```python
from build123d import *

# Parameters (mm, degrees)
SKETCH1_W           = 250
SKETCH1_H           = 62.9
BOSS_EXTRUDE1_DEPTH = 3
SKETCH3_W           = 3
SKETCH3_H           = 20
CUT_EXTRUDE1_DEPTH  = 258.808863308
CUT_EXTRUDE2_REACH  = 259.809
SKETCH4_W           = 20
SKETCH4_H           = 3
CUT_EXTRUDE3_REACH  = 259.809
SKETCH5_W           = 20
SKETCH5_H           = 3
CUT_EXTRUDE4_REACH  = 259.809
SKETCH6_W           = 90
SKETCH6_H           = 3


with BuildPart() as part:
    # Sketch1 → Boss-Extrude1 (new body)
    with BuildSketch(Plane(origin=(0, 0, 0), x_dir=(1, 0, 0), z_dir=(0, 1, 0))):
        with Locations((125, 31.45)):
            Rectangle(SKETCH1_W, SKETCH1_H)
    extrude(amount=BOSS_EXTRUDE1_DEPTH)

    # Sketch3 → Cut-Extrude1 (cut, through all)
    with BuildSketch(Plane(origin=(0, 3, 0), x_dir=(1, 0, 0), z_dir=(0, 1, 0))):
        with Locations((1.5, 32.9)):
            Rectangle(SKETCH3_W, SKETCH3_H)
        with Locations((248.5, 32.9)):
            Rectangle(SKETCH3_W, SKETCH3_H)
    extrude(amount=-CUT_EXTRUDE1_DEPTH, mode=Mode.SUBTRACT)

    # Sketch4 → Cut-Extrude2 (cut, up to next)
    with BuildSketch(Plane(origin=(0, 3, 0), x_dir=(1, 0, 0), z_dir=(0, 1, 0)), mode=Mode.PRIVATE) as cut_extrude2_sk1:
        with Locations((10, 61.4)):
            Rectangle(SKETCH4_W, SKETCH4_H)
    cut_extrude2_tool1 = extrude(cut_extrude2_sk1.sketch, amount=-CUT_EXTRUDE2_REACH, mode=Mode.PRIVATE) & part.part
    add(cut_extrude2_tool1.solids().sort_by_distance((10, 3, -61.4))[0], mode=Mode.SUBTRACT)

    # Sketch5 → Cut-Extrude3 (cut, up to next)
    with BuildSketch(Plane(origin=(0, 3, 0), x_dir=(1, 0, 0), z_dir=(0, 1, 0)), mode=Mode.PRIVATE) as cut_extrude3_sk1:
        with Locations((240, 61.4)):
            Rectangle(SKETCH5_W, SKETCH5_H)
    cut_extrude3_tool1 = extrude(cut_extrude3_sk1.sketch, amount=-CUT_EXTRUDE3_REACH, mode=Mode.PRIVATE) & part.part
    add(cut_extrude3_tool1.solids().sort_by_distance((240, 3, -61.4))[0], mode=Mode.SUBTRACT)

    # Sketch6 → Cut-Extrude4 (cut, up to next)
    with BuildSketch(Plane(origin=(0, 3, 0), x_dir=(1, 0, 0), z_dir=(0, 1, 0)), mode=Mode.PRIVATE) as cut_extrude4_sk1:
        with Locations((125, 61.4)):
            Rectangle(SKETCH6_W, SKETCH6_H)
    cut_extrude4_tool1 = extrude(cut_extrude4_sk1.sketch, amount=-CUT_EXTRUDE4_REACH, mode=Mode.PRIVATE) & part.part
    add(cut_extrude4_tool1.solids().sort_by_distance((125, 3, -61.4))[0], mode=Mode.SUBTRACT)


solid = part.part
```
Here's how the part is built. I have some questions about the finished solid (model axes, mm). Round coordinates to 2 decimals unless told otherwise and drop trailing zeros. Order: outer loops, then holes, each group sorted by start corner. A loop starts at its lowest first (then second) coordinate and runs counter-clockwise, first axis right, second up. Notation, with made-up numbers: M 44.5,35 L 51.5,35 A30 ccw 51.5,71 Z; hole C 69,51.25 d1. An arc over 180 degrees is marked long. One line per question, with ' | ' between items.
1) For pin 1 Ø0.9 at (y, z) = (1, -61) entering from -X; pin 2 Ø1.5 at (y, z) = (2, -60.5) entering from +X; pin 3 Ø1.5 at (y, z) = (1, -61.5) entering from +X; pin 4 Ø1.5 at (x, y) = (6, 2) entering from -Z, each with a flat end and sliding along its axis, tell me the tip position at first contact or that it passes through.
Working result:
pin 1: x = 20 | pin 2: x = 250 | pin 3: x = 230 | pin 4: z = -59.9
2) I want a section at C-C, the plane z = -33. Write out the boundary of the cut face in (x, y), then the cut area to 3 significant figures.
Working result:
outline: M 3,0 L 247,0 L 247,3 L 3,3 Z | area: 732 mm²
3) I need wall thicknesses on line 1 along Z through (x, y) = (143.5, 2.4); line 2 along X through (y, z) = (1.75, -38.5). Which ranges of each line are inside material? Lowest first, please.
Working result:
line 1: -59.9 to 0 | line 2: 3 to 247
4) I want a section at A-A, the plane y = 1.05. Write out the boundary of the cut face in (x, z), then the cut area to 3 significant figures.
Working result:
outline: M 0,-59.9 L 20,-59.9 L 20,-62.9 L 80,-62.9 L 80,-59.9 L 170,-59.9 L 170,-62.9 L 230,-62.9 L 230,-59.9 L 250,-59.9 L 250,-42.9 L 247,-42.9 L 247,-22.9 L 250,-22.9 L 250,0 L 0,0 L 0,-22.9 L 3,-22.9 L 3,-42.9 L 0,-42.9 Z | area: 15,200 mm²
5) I want a section at B-B, the plane x = 149.5. Write out the boundary of the cut face in (y, z).
Working result:
outline: M 0,-59.9 L 3,-59.9 L 3,0 L 0,0 Z
